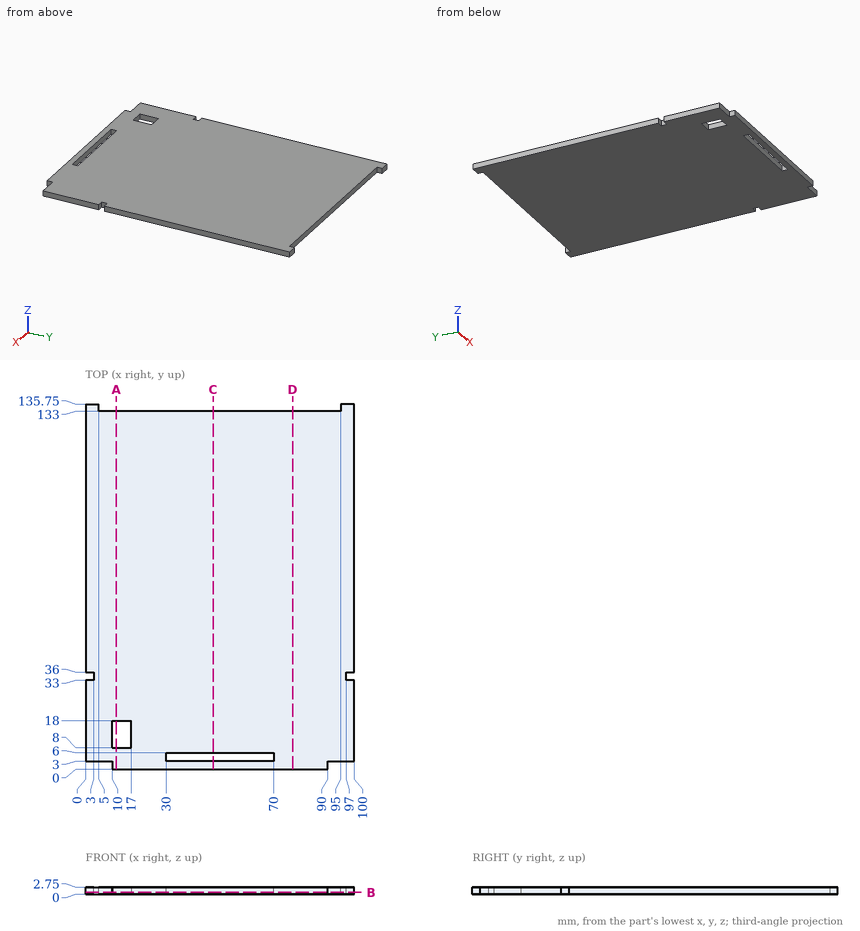
Verification items for this drawing (mm, ordinates from the low corner). Round coordinates to 2 decimals unless told otherwise and drop trailing zeros. Order: outer loops, then holes, each group sorted by start corner. A loop starts at its lowest first (then second) coordinate and runs counter-clockwise, first axis right, second up. Notation, with made-up numbers: M -29,72.5 L -3,72.5 A21 cw -3,79.5 Z; hole C 18.5,-29.5 d1. An arc over 180 degrees is marked long. Answer in a Markdown table with one row per item. Add a question column.
Item 1: Sectioned sample at C-C, the plane x = 47.5. Enter the section's corners in (y, z).
Item 2: Sectioned sample at D-D, the plane x = 77. Enter the section's corners in (y, z), plus the area to 3 significant figures.
Item 3: Material ranges on L1, parallel to Y at x = 16, z = 1.95; L2, parallel to Y at x = 30.5, z = 1.7; L3, parallel to Y at x = 74, z = 1.2, recorded low to high. Write a range as [from, to].
Item 4: Sectioned sample at B-B, the plane z = 0.8. Enter the section's corners in (x, y), plus the area to 3 significant figures.
Item 5: Sectioned sample at A-A, the plane x = 11.5. Enter the section's corners in (y, z), plus the area to 3 significant figures.
Item 6: Depth check by flat-ended pin: pin 1 Ø1.4 at (x, z) = (99, 1.5) entering from -Y. Enter the tip coordinate at first touch or a pass-through.
Filled in:
| question | item | result |
|---|---|---|
| 1 | outline | M 0,0 L 3,0 L 3,2.75 L 0,2.75 Z; M 6,0 L 133,0 L 133,2.75 L 6,2.75 Z |
| 2 | outline | M 0,0 L 133,0 L 133,2.75 L 0,2.75 Z |
| 2 | area | 366 mm² |
| 3 | L1 | y = [0, 8], [18, 133] |
| 3 | L2 | y = [0, 3], [6, 133] |
| 3 | L3 | y = [0, 133] |
| 4 | outline | M 0,3 L 10,3 L 10,0 L 90,0 L 90,3 L 100,3 L 100,33 L 97,33 L 97,36 L 100,36 L 100,135.75 L 95,135.75 L 95,133 L 5,133 L 5,135.75 L 0,135.75 L 0,36 L 3,36 L 3,33 L 0,33 Z; hole M 10,8 L 17,8 L 17,18 L 10,18 Z; hole M 30,3 L 70,3 L 70,6 L 30,6 Z |
| 4 | area | 13,100 mm² |
| 5 | outline | M 0,0 L 8,0 L 8,2.75 L 0,2.75 Z; M 18,0 L 133,0 L 133,2.75 L 18,2.75 Z |
| 5 | area | 338 mm² |
| 6 | pin 1 | stops at y = 3 |
